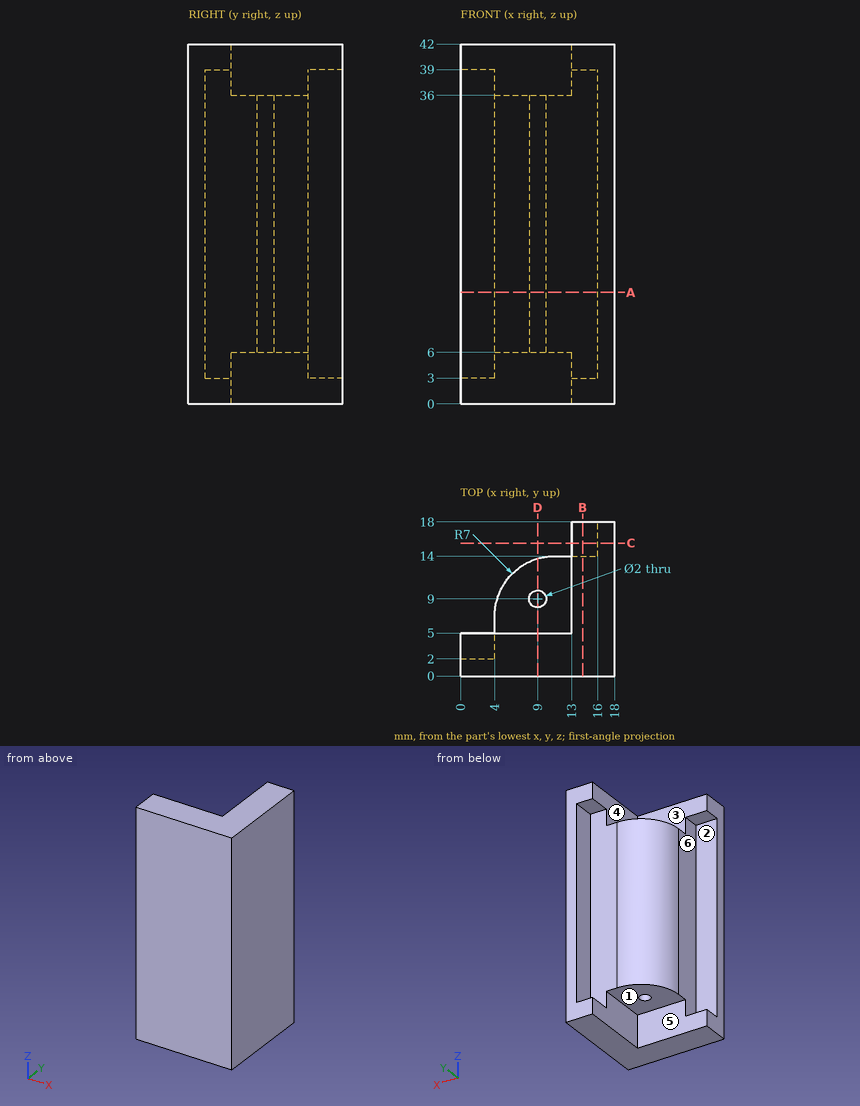
Source: three-view drawing plus pictorial views. Frame: mm from the lowest corner of the part. A direction names the side the tool comes from. Give positions to 0.01 mm unless a question says otherwise; leave off trailing zeros. Order: outer loops, then holes, each group sorted by start corner. A loop starts at its lowest first (then second) coordinate and runs counter-clockwise, first axis right, second up. Notation, with made-up numbers: (-11.5, 45) - (20.5, 45) arc R22 ccw to (20.5, 58) - close; hole circle Ø6 at (11.25, -16). An arc over 180 degrees is marked (long way). Answer as a JSON object with one key per item and string values. Group by question number.
Q1. Set-up query: the marked faces 4, 5 and 6. Return all of +Z, -Z, +X, -X, +Y, -Y with unobstructed straight access to the full face (end or side cutting, diameter ignored); none if empty.
Q2. Line query: probe 1 along Y at (x, z) = (3.5, 7); probe 2 along Z at (x, y) = (9, 7.75); probe 3 along Y at (x, z) = (9, 28). Output: solid intervals per line, ascending.
Q3. Mould query, pull axis Z, two halves, no side actions, for the marked faces 1, 2 and 3. Classes: pulls with the +Z half, pulls with the -Z half, needs draft (parallel to the pull), parting line crosses it, or undercut.
Q4. First-contact query: pin 1 Ø2 at (x, z) = (1, 29.5) entering from +Y; pin 2 Ø3 at (y, z) = (13, 39.5) entering from -X; pin 3 Ø3 at (x, z) = (8, 39.5) entering from +Y. Flat tips, straight axial feed; report the tip coordinate or a pass-through.
Q5. Cut plane A-A, the plane z = 13. Output: boundary loops of the cut face in (x, y).
Q6. Cut plane D-D, the plane x = 9. Output: boundary loops of the cut face in (y, z).
Q7. Cut plane C-C, the plane y = 15.5. Output: boundary loops of the cut face in (x, z), then the cut area to 3 significant figures.
Q8. Cut plane B-B, the plane x = 14.25. Output: boundary loops of the cut face in (y, z), then the cut area to 3 significant figures.
Results:
{
 "1": {"face 4": "+Z, -X, +Y", "face 5": "-Z, -X, +Y", "face 6": "-X, +Y"},
 "2": {"probe 1": "0 to 2", "probe 2": "6 to 36", "probe 3": "0 to 8, 10 to 13.71"},
 "3": {"face 1": "pulls with the -Z half", "face 2": "undercut", "face 3": "needs draft"},
 "4": {"pin 1": "y = 2", "pin 2": "x = 13", "pin 3": "y = 5"},
 "5": {"outline": "(0, 0) - (18, 0) - (18, 18) - (16, 18) - (16, 14) - (11, 14) arc R7 ccw to (4, 7) - (4, 2) - (0, 2) - close; hole circle Ø2 at (9, 9)"},
 "6": {"outline": "(0, 0) - (5, 0) - (5, 6) - (8, 6) - (8, 36) - (5, 36) - (5, 42) - (0, 42) - close; (10, 6) - (13.71, 6) - (13.71, 36) - (10, 36) - close"},
 "7": {"outline": "(13, 0) - (18, 0) - (18, 42) - (13, 42) - (13, 39) - (16, 39) - (16, 3) - (13, 3) - close", "area": "102 mm^2"},
 "8": {"outline": "(0, 0) - (18, 0) - (18, 3) - (14, 3) - (14, 39) - (18, 39) - (18, 42) - (0, 42) - close", "area": "612 mm^2"}
}
